Verification items for the finished model (mm, model axes). Face numbers are marked on the shaded views. Give positions to 0.01 mm unless a question says otherwise; leave off trailing zeros. Loops run counter-clockwise (first coordinate to the right, second up) from the corner with the lowest first, then second, coordinate; pieces in that order, holes last. Notation, with made-up numbers: (13, -4.5) -> (35, -4.5) arc R27 cw to (35, 20.5) -> close; hole circle Ø10 at (-26, 6). An arc over 180 degrees is marked (long way). Use one line per item in the form item = value. Start each with the question number.
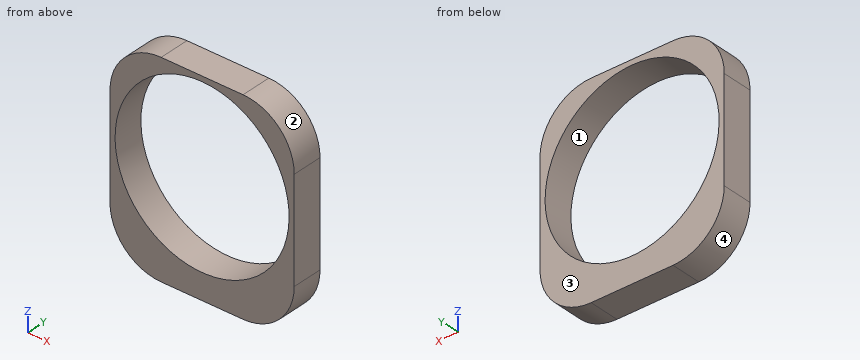
from build123d import *

# Parameters (mm, degrees)
SKETCH1_W           = 180
SKETCH1_H           = 200
BOSS_EXTRUDE1_DEPTH = 30
SKETCH7_R           = 85
CUT_EXTRUDE1_DEPTH  = 40
FILLET1_R           = 50
FILLET2_R           = 50
FILLET3_R           = 50
FILLET4_R           = 50


with BuildPart() as part:
    # Sketch1 → Boss-Extrude1 (new body)
    with BuildSketch(Plane(origin=(0, 0, 0), x_dir=(1, 0, 0), z_dir=(0, 1, 0))):
        with Locations((-90, 100)):
            Rectangle(SKETCH1_W, SKETCH1_H)
    extrude(amount=BOSS_EXTRUDE1_DEPTH)

    # Sketch7 → Cut-Extrude1 (cut)
    with BuildSketch(Plane(origin=(0, 30, 0), x_dir=(1, 0, 0), z_dir=(0, 1, 0))):
        with Locations(Location((-90, 90, 0), (0, 0, 270))):
            Circle(SKETCH7_R)
    extrude(amount=-CUT_EXTRUDE1_DEPTH, mode=Mode.SUBTRACT)

    # Fillet1
    fillet1_edges = [part.edges().sort_by_distance(p)[0] for p in [
        (0, 15, -200),
    ]]
    fillet(fillet1_edges, radius=FILLET1_R)

    # Fillet2
    fillet2_edges = [part.edges().sort_by_distance(p)[0] for p in [
        (0, 15, 0),
    ]]
    fillet(fillet2_edges, radius=FILLET2_R)

    # Fillet3
    fillet3_edges = [part.edges().sort_by_distance(p)[0] for p in [
        (-180, 15, 0),
    ]]
    fillet(fillet3_edges, radius=FILLET3_R)

    # Fillet4
    fillet4_edges = [part.edges().sort_by_distance(p)[0] for p in [
        (-180, 15, -200),
    ]]
    fillet(fillet4_edges, radius=FILLET4_R)


solid = part.part
Item 1: Sectioned sample at A-A, the plane z = -90. Enter the section's corners in (x, y).
Item 2: Sectioned sample at C-C, the plane y = 21.5. Enter the section's corners in (x, z), and give its area (3 significant figures).
Item 3: Sectioned sample at B-B, the plane x = -90. Enter the section's corners in (y, z).
Item 4: Material ranges on line 1 (X direction, y = 18, z = -90); line 2 (X direction, y = 13.25, z = -83.5); line 3 (Z direction, x = -124, y = 6.5), recorded low to high.
Item 5: Draft check along X on the marked faces 1, 2, 3 and 4. Enter one of: +X half, -X half, draft (parallel to the pull), parting line (faces both ways), or undercut.
Item 6: Gauge pin test, flat end, axial feed: pin 1 Ø6 at (x, y) = (-146.5, 15) entering from +Z. Record the tip position at first contact, or that the pin passes through.
Outcome:
q1.outline = (-180, 0) -> (-175, 0) -> (-175, 30) -> (-180, 30) -> close; (-5, 0) -> (0, 0) -> (0, 30) -> (-5, 30) -> close
q2.outline = (-180, -150) arc R50 ccw to (-130, -200) -> (-50, -200) arc R50 ccw to (0, -150) -> (0, -50) arc R50 ccw to (-50, 0) -> (-130, 0) arc R50 ccw to (-180, -50) -> close; hole circle Ø170 at (-90, -90)
q2.area = 11,200 mm^2
q3.outline = (0, -200) -> (30, -200) -> (30, -175) -> (0, -175) -> close; (0, -5) -> (30, -5) -> (30, 0) -> (0, 0) -> close
q4.line_1 = -180 to -175, -5 to 0
q4.line_2 = -180 to -174.75, -5.25 to 0
q4.line_3 = -200 to -167.9, -12.1 to 0
q5.face_1 = undercut
q5.face_2 = +X half
q5.face_3 = draft
q5.face_4 = -X half
q6.pin_1 = -1.86
